from build123d import *

# Parameters (mm, degrees)
SKETCH1_W           = 10
SKETCH1_H           = 5
BOSS_EXTRUDE1_DEPTH = 2.5


with BuildPart() as part:
    # Sketch1 → Boss-Extrude1 (new, symmetric)
    with BuildSketch(Plane.XY):
        with BuildLine():
            ThreePointArc((95.875, 0), (91.225320151, 11.225320151), (80, 15.875))
            Line((80, 15.875), (-80, 15.875))
            ThreePointArc((-80, 15.875), (-91.225320151, 11.225320151), (-95.875, 0))
            Line((-95.875, 0), (-95.875, 30))
            Line((-95.875, 30), (95.875, 30))
            Line((95.875, 30), (95.875, 0))
        make_face()
        with Locations((-60, 32.5)):
            Rectangle(SKETCH1_W, SKETCH1_H)
        with Locations((0, 32.5)):
            Rectangle(SKETCH1_W, SKETCH1_H)
        with Locations((60, 32.5)):
            Rectangle(SKETCH1_W, SKETCH1_H)
    extrude(amount=BOSS_EXTRUDE1_DEPTH, both=True)


solid = part.part
Verification items for the finished model (mm, model axes). A direction names the side the tool comes from. Coordinates: 2 decimals unless noted, no trailing zeros. Write each loop counter-clockwise with the first axis right and the second up, starting at its lowest first coordinate (ties: lowest second). Pieces come first, ordered by that corner, then holes. Notation, with made-up numbers: M 61.5,18.5 L 96.5,18.5 A28 ccw 96.5,37.5 Z; hole C 58,40 d7. An arc over 180 degrees is marked long. Use a Markdown table: item, result.
Q1. Sectioned sample at B-B, the plane z = -0.6. Record the boundary of the cut face in (x, y) (3 decimals).
Reply:
| item | result |
|---|---|
| outline | M -95.875,0 A15.875 cw -80,15.875 L 80,15.875 A15.875 cw 95.875,0 L 95.875,30 L 65,30 L 65,35 L 55,35 L 55,30 L 5,30 L 5,35 L -5,35 L -5,30 L -55,30 L -55,35 L -65,35 L -65,30 L -95.875,30 Z |
Q2. Go/stop test with flat-tipped pins: P1, Ø1.5, axis at x = 28.5, z = 0.5, coming from the +Y side; P2, Ø1.5, axis at x = 9, z = 0, coming from the -Y side (3 decimals); P3, Ø2.5, axis at y = 32.5, z = 0.5, coming from the -X side; P4, Ø2, axis at x = 22, y = 31.5, coming from the +Z side. Record where each tip stops, or that it passes through.
Reply:
| item | result |
|---|---|
| P1 | stops at y = 30 |
| P2 | stops at y = 15.875 |
| P3 | stops at x = -65 |
| P4 | passes through |
Q3. Draft check along X on faces 5 (the face through (80, 30, 0)), 6 (the face through (-65, 32, 0)), 7 (the face through (55, 32, 0)), 8 (the face through (95.875, 15, 0)). Enter one of: +X half, -X half, draft (parallel to the pull), parting line (faces both ways), or undercut.
Reply:
| item | result |
|---|---|
| face 5 | draft |
| face 6 | -X half |
| face 7 | undercut |
| face 8 | +X half |
Q4. Set-up check for faces 1 (the face through (65, 32, 0)), 2 (the face through (-30, 30, 0)), 3 (the face through (-81, 30, 0)), 4 (the face through (-91.1, 11.35, 0.04)): record each of +Z, -Z, +X, -X, +Y, -Y from which the full face is reachable in a straight line by a thin tool's end or side.
Reply:
| item | result |
|---|---|
| face 1 | +Z, -Z, +X, +Y |
| face 2 | +Z, -Z, +Y |
| face 3 | +Z, -Z, -X, +Y |
| face 4 | +Z, -Z, -Y |
Q5. Sectioned sample at A-A, the plane y = 7. Record the boundary of the cut face in (x, z) (3 decimals).
Reply:
| item | result |
|---|---|
| outline | M -95.875,-2.5 L -94.248,-2.5 L -94.248,2.5 L -95.875,2.5 Z; M 94.248,-2.5 L 95.875,-2.5 L 95.875,2.5 L 94.248,2.5 Z |
Q6. Thickness scan on line 1 (Y direction, x = -63, z = -1.35) (3 decimals); line 2 (Y direction, x = 31.5, z = 1.15) (3 decimals); line 3 (X direction, y = 10.5, z = 1.2) (3 decimals). Record the ranges inside material, lowest first.
Reply:
| item | result |
|---|---|
| line 1 | y = 15.875 to 35 |
| line 2 | y = 15.875 to 30 |
| line 3 | x = -95.875 to -91.907, 91.907 to 95.875 |
Q7. Sectioned sample at C-C, the plane x = -37.5. Record the boundary of the cut face in (y, z) (3 decimals).
Reply:
| item | result |
|---|---|
| outline | M 15.875,-2.5 L 30,-2.5 L 30,2.5 L 15.875,2.5 Z |
